Build history of the part. All positions in model axes, mm. A direction names the side the tool comes from. Round coordinates to 2 decimals unless told otherwise and drop trailing zeros. Write each loop counter-clockwise with the first axis right and the second up, starting at its lowest first coordinate (ties: lowest second). Pieces come first, ordered by that corner, then holes. Notation, with made-up numbers: (3.5, -16) - (30.5, -16) arc R8 cw to (30.5, -4) - close; hole circle Ø2 at (79, 10). An arc over 180 degrees is marked (long way). Write each question's results on one line, items separated by ' | '.
from build123d import *

# Parameters (mm, degrees)
BOSS_EXTRU_1_DEPTH      = 285
ENL_V_MAT_EXTRU_1_DEPTH = 543.56
ESQUISSE4_W             = 6.35
ESQUISSE4_H             = 25.4
BOSS_EXTRU_2_DEPTH      = 95.25


with BuildPart() as part:
    # Esquisse1 → Boss.-Extru.1 (new, symmetric)
    with BuildSketch(Plane.XY):
        Polygon((-29.9, -288.29), (131.5, -161.29), (131.5, 288.29), (-131.5, 288.29), (-131.5, -288.29), (-36.25, -288.29), (-36.25, -313.69), (-29.9, -313.69), align=None)
    extrude(amount=BOSS_EXTRU_1_DEPTH, both=True)

    # Esquisse2 → Enlèv. mat.-Extru.1 (cut)
    with BuildSketch(Plane.XY.offset(272.3)):
        Polygon((-125.15, 288.29), (-125.15, -288.29), (-40.168758445, -288.29), (125.15, -158.206466403), (125.15, 288.29), align=None)
    extrude(amount=-ENL_V_MAT_EXTRU_1_DEPTH, mode=Mode.SUBTRACT)

    # Esquisse4 → Boss.-Extru.2 (add)
    with BuildSketch(Plane.ZY.offset(36.25)):
        with Locations((-281.825, -300.99)):
            Rectangle(ESQUISSE4_W, ESQUISSE4_H)
    boss_extru_2 = extrude(amount=BOSS_EXTRU_2_DEPTH)

    # Symétrie1: Boss.-Extru.2 across plane
    add(boss_extru_2.mirror(Plane.XY))


solid = part.part
(1) Slice it at D-D, the plane x = -3.5. Write the cut outline in (y, z).
Worked answers:
outline: (-267.52, -285) - (288.29, -285) - (288.29, -271.26) - (-259.44, -271.26) - (-259.44, 272.3) - (288.29, 272.3) - (288.29, 285) - (-267.52, 285) - close
(2) Flat gauge pins, fed straight in: pin 1 Ø6 at (x, z) = (103, 91) entering from +Y; pin 2 Ø1 at (x, z) = (71, -35) entering from -Y; pin 3 Ø1.5 at (x, z) = (67.5, -158) entering from -Y. Where does each tip first touch, or does it go through?
Worked answers:
pin 1: stops at y = -173.27 | pin 2: stops at y = -209.29 | pin 3: stops at y = -212.24
(3) Slice it at B-B, the plane y = 18. Write the cut outline in (x, z).
Worked answers:
outline: (-131.5, -285) - (131.5, -285) - (131.5, 285) - (-131.5, 285) - close; hole (-125.15, -271.26) - (125.15, -271.26) - (125.15, 272.3) - (-125.15, 272.3) - close
(4) Two-plate mould, pull along X, no slides. Class faces 1 (the flat face through (-29.9, -301, 4)), 2 (the flat face through (-125.15, 4, 4)), 3 (the flat face through (-83, -301, 278.65)), 4 (the flat face through (-2, 4, -271.26)): released by +X, released by -X, zero draft, split by the parting line, or undercut.
Worked answers:
face 1: released by +X | face 2: undercut | face 3: zero draft | face 4: undercut
(5) Slice it at A-A, the plane x = -71. Write the cut outline in (y, z).
Worked answers:
outline: (-313.69, -285) - (288.29, -285) - (288.29, -271.26) - (-288.29, -271.26) - (-288.29, -278.65) - (-313.69, -278.65) - close; (-313.69, 278.65) - (-288.29, 278.65) - (-288.29, 272.3) - (288.29, 272.3) - (288.29, 285) - (-313.69, 285) - close
(6) Drill centre lines: probe 1 along X at (y, z) = (-55, 78.5); probe 2 along Z at (x, y) = (-39, -115.5); probe 3 along X at (y, z) = (-273.5, -14.5). Where is each one in solid material? Low to high. Write a range as [from, to].
Worked answers:
probe 1: x = [-131.5, -125.15], [125.15, 131.5] | probe 2: z = [-285, -271.26], [272.3, 285] | probe 3: x = [-131.5, -125.15], [-21.37, -11.1]
(7) Tool access for faces 5 (the flat face through (2, -17, -285)), 6 (the flat face through (41.33, -224.16, 4.32)), 7 (the flat face through (-36.25, -301, 4)): list every direction of +Z, -Z, +X, -X, +Y, -Y with a clear straight run to the whole face (end or side of a thin tool).
Worked answers:
face 5: -Z, +X, -X, +Y, -Y | face 6: +Y | face 7: -X, -Y
(8) Slice it at C-C, the plane z = -29. Write the cut outline in (x, y).
Worked answers:
outline: (-131.5, -288.29) - (-125.15, -288.29) - (-125.15, 288.29) - (-131.5, 288.29) - close; (-40.17, -288.29) - (-36.25, -288.29) - (-36.25, -313.69) - (-29.9, -313.69) - (-29.9, -288.29) - (131.5, -161.29) - (131.5, 288.29) - (125.15, 288.29) - (125.15, -158.21) - close
